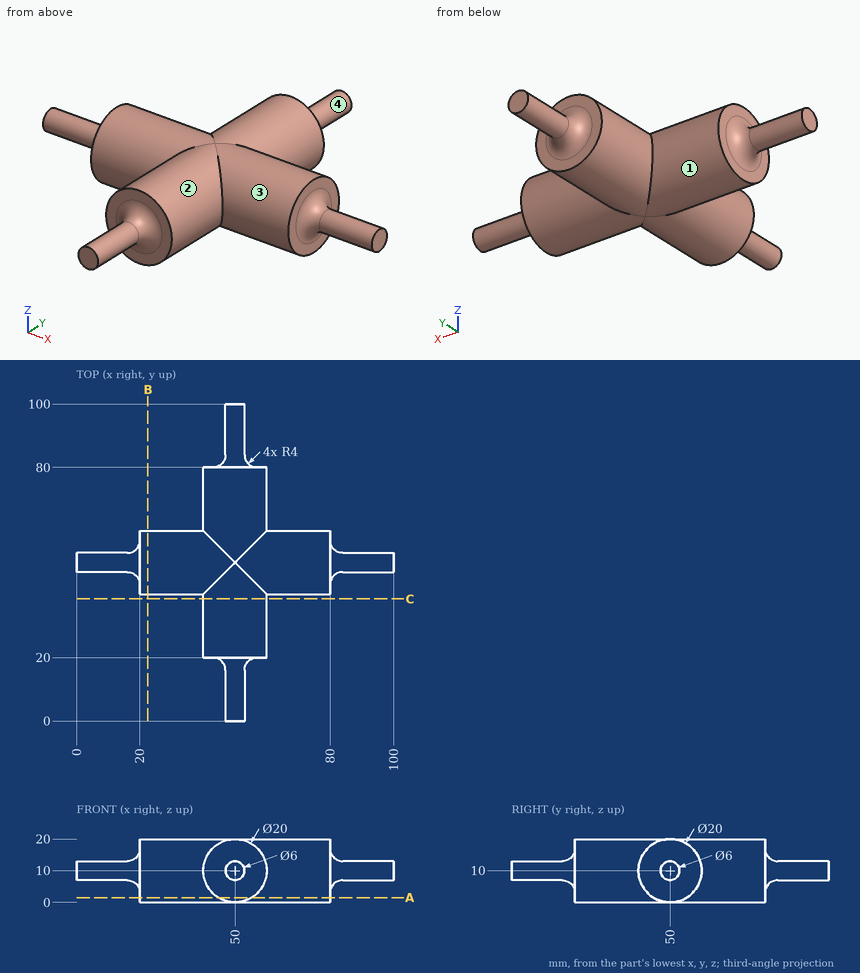
Can you work these out from the drawing? Everything is in mm from the part's minimum corner. A direction names the side the tool comes from. Give positions to 0.01 mm unless a question says otherwise; leave off trailing zeros. Loops run counter-clockwise (first coordinate to the right, second up) from the corner with the lowest first, then second, coordinate; pieces in that order, holes last. Notation, with made-up numbers: M 39,54 L 43,54 A16 ccw 43,66 Z; hole C -13.5,48 d11. An arc over 180 degrees is marked long. Use CSV: the item, a comma, the result in double quotes. Start each with the question number.
1. On a 3-axis mill with a long thin cutter (end or side, diameter ignored), from which of +Z, -Z, +X, -X, +Y, -Y can I reach the whole of each face in a straight line? I mean the marked faces 1, 2, 3 and 4. Say none if no direction works.
2. If I drill on L1, parallel to Z at x = 49.5, y = 47.5; L2, parallel to Y at x = 54, z = 2.5; L3, parallel to Y at x = 62, z = 9.75, over which ranges is the centre line in solid material (lowest first)?
3. Imagine slicing it at A-A, the plane z = 1.5. Write out the boundary of the cut face in (x, y), plus the area to 3 significant figures.
4. Imagine slicing it at B-B, the plane x = 22.5. Write out the boundary of the cut face in (y, z), plus the area to 3 significant figures.
5. For P1, Ø1.5, axis at y = 41, z = 4, coming from the +X side; P2, Ø1.5, axis at y = 80, z = 15, coming from the +X side; P3, Ø6, axis at x = 39, z = 10, coming from the +Y side, each with a flat end and sliding along its axis, tell me the tip position at first contact or that it passes through.
Response values:
1,face 1,"-X"
1,face 2,"-Y"
1,face 3,"+X"
1,face 4,"+Y"
2,L1,"0.01 to 19.99"
2,L2,"20 to 80"
2,L3,"40 to 60"
3,outline,"M 20,44.73 L 44.73,44.73 L 44.73,20 L 55.27,20 L 55.27,44.73 L 80,44.73 L 80,55.27 L 55.27,55.27 L 55.27,80 L 44.73,80 L 44.73,55.27 L 20,55.27 Z"
3,area,"1,150 mm^2"
4,outline,"C 50,10 d20"
4,area,"314 mm^2"
5,P1,"x = 58.51"
5,P2,"x = 59.05"
5,P3,"y = 80"
